Can you work these out from the model? Positions are in its coordinate system, mm. Round coordinates to 2 decimals unless told otherwise and drop trailing zeros. Loops run counter-clockwise (first coordinate to the right, second up) from the corner with the lowest first, then second, coordinate; pieces in that order, holes last. Notation, with made-up numbers: M -34.75,69 L 24.25,69 A12 ccw 24.25,73 Z; hole C -23.5,-21 d9. An arc over 180 degrees is marked long. Answer as CSV lines item,"result".
from build123d import *

# Parameters (mm, degrees)
SKETCH001_R   = 2.5
SKETCH001_R_2 = 5
SKETCH001_R_3 = 2
PAD_DEPTH     = 12


with BuildPart() as part:
    # Sketch001 → Pad (new body)
    with BuildSketch(Plane(origin=(0, 0, 0), x_dir=(1, 0, 0), z_dir=(0, 0, -1))):
        with BuildLine():
            Line((-96.421355, 48.651027), (96.421355, 48.651027))
            ThreePointArc((96.421355, -48.651027), (108, 0), (96.421355, 48.651027))
            Line((96.421355, -48.651027), (-96.421355, -48.651027))
            ThreePointArc((-96.421355, 48.651027), (-108, 0), (-96.421355, -48.651027))
        make_face()
        with Locations((93.311833, 38.651027)):
            Circle(SKETCH001_R, mode=Mode.SUBTRACT)
        with Locations((93.311833, -38.651027)):
            Circle(SKETCH001_R, mode=Mode.SUBTRACT)
        with Locations((-93.311833, 38.651027)):
            Circle(SKETCH001_R, mode=Mode.SUBTRACT)
        with Locations((-93.311833, -38.651027)):
            Circle(SKETCH001_R, mode=Mode.SUBTRACT)
        with Locations((-45, 0)):
            Circle(SKETCH001_R_2, mode=Mode.SUBTRACT)
        with Locations((45, 0)):
            Circle(SKETCH001_R_2, mode=Mode.SUBTRACT)
        with Locations((54.75, 16.887495)):
            Circle(SKETCH001_R, mode=Mode.SUBTRACT)
        with Locations((25.5, 0)):
            Circle(SKETCH001_R, mode=Mode.SUBTRACT)
        with Locations((54.75, -16.887495)):
            Circle(SKETCH001_R, mode=Mode.SUBTRACT)
        with Locations((-54.75, 16.887495)):
            Circle(SKETCH001_R, mode=Mode.SUBTRACT)
        with Locations((-25.5, 0)):
            Circle(SKETCH001_R, mode=Mode.SUBTRACT)
        with Locations((-54.75, -16.887495)):
            Circle(SKETCH001_R, mode=Mode.SUBTRACT)
        Circle(SKETCH001_R_3, mode=Mode.SUBTRACT)
    extrude(amount=PAD_DEPTH)


solid = part.part
Item 1: If we section it at D-D on x = 25.5: Write out the boundary of the cut face in (y, z), then the cut area to 3 significant figures.
Output:
outline,"M -48.65,-12 L -2.5,-12 L -2.5,0 L -48.65,0 Z; M 2.5,-12 L 48.65,-12 L 48.65,0 L 2.5,0 Z"
area,"1,110 mm2"
Item 2: If we section it at C-C on z = -5: State how many separate pieces and enclosed holes the cut face has, then the cut area to 3 significant figures.
Output:
separate pieces,"1"
enclosed holes,"13"
area,"19,900 mm2"
Item 3: If we section it at A-A on y = 0: Write out the boundary of the cut face in (x, z), then the cut area to 3 significant figures.
Output:
outline,"M -108,-12 L -50,-12 L -50,0 L -108,0 Z; M -40,-12 L -28,-12 L -28,0 L -40,0 Z; M -23,-12 L -2,-12 L -2,0 L -23,0 Z; M 2,-12 L 23,-12 L 23,0 L 2,0 Z; M 28,-12 L 40,-12 L 40,0 L 28,0 Z; M 50,-12 L 108,-12 L 108,0 L 50,0 Z"
area,"2,180 mm2"
Item 4: We'd pull the mould along Y, two halves only. Please class faces 1 (the face through (-107.998, -0.707, -5.916)), 2 (the face through (2, -11, 0)), 3 (the face through (-50, 0, -6)): released by +Y, released by -Y, zero draft, split by the parting line, or undercut.
Output:
face 1,"split by the parting line"
face 2,"zero draft"
face 3,"undercut"
Item 5: If we section it at B-B on x = -45: Write out the boundary of the cut face in (y, z), then the cut area to 3 significant figures.
Output:
outline,"M -48.65,-12 L -5,-12 L -5,0 L -48.65,0 Z; M 5,-12 L 48.65,-12 L 48.65,0 L 5,0 Z"
area,"1,050 mm2"
Item 6: Will these pins go through, and if not, where does the flat tip stop? pin 1 (4.5 mm diameter, centred on x = -54.75, y = -16.89, fed in from +Z); pin 2 (2 mm diameter, centred on y = 25, z = -4.5, fed in from -X); pin 3 (3 mm diameter, centred on y = -27, z = -9.5, fed in from +X); pin 4 (2 mm diameter, centred on y = -26, z = -3, fed in from +X).
Output:
pin 1,"passes through"
pin 2,"stops at x = -105.3"
pin 3,"stops at x = 104.95"
pin 4,"stops at x = 105.07"
Item 7: If I drill on line 1 along Y through (x, z) = (-54.75, -4.5); line 2 along X through (y, z) = (15.5, -7); line 3 along X through (y, z) = (-36.5, -8.75), over which ranges is the centre line in solid material (lowest first)? Write a range as from..to.
Output:
line 1,"y = -48.65..-19.39, -14.39..14.39, 19.39..48.65"
line 2,"x = -106.88..-56.83, -52.67..52.67, 56.83..106.88"
line 3,"x = -101.65..-94.59, -92.04..92.04, 94.59..101.65"
